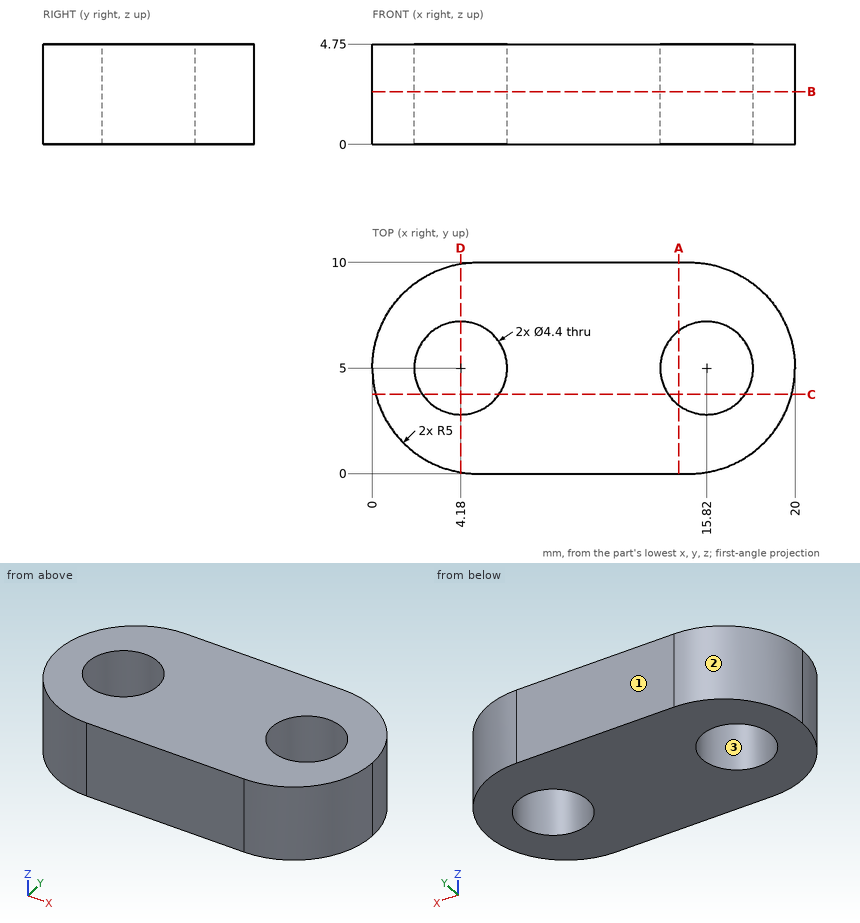
Here's the drawing with two shaded views (mm, measured from the low corner). I have some questions. Round coordinates to 2 decimals unless told otherwise and drop trailing zeros. Write each loop counter-clockwise with the first axis right and the second up, starting at its lowest first coordinate (ties: lowest second). Pieces come first, ordered by that corner, then holes. Notation, with made-up numbers: M 23,-28.75 L 59,-28.75 A28 cw 59,1.25 Z; hole C 41,61.5 d6. An arc over 180 degrees is marked long. Answer in a Markdown table with one row per item. Add a question column.
Q1. Imagine slicing it at B-B (z = 2.5). Give the number of separate pieces and of enclosed holes in the cut face, then the cut area to 3 significant figures.
Q2. If we mould it in two halves opening along X, with no side actions, what happens to the marked faces 1, 2 and 3? For each: +X half, -X half, draft (parallel to the pull), parting line (faces both ways), or undercut.
Q3. Imagine slicing it at A-A (x = 14.5). Please give me the cut outline in (y, z), then the cut area to 3 significant figures.
Q4. If I drill on line 1 (X direction, y = 6, z = 0.55); line 2 (X direction, y = 3.25, z = 2.9); line 3 (Y direction, x = 15.82, z = 3), over which ranges is the centre line in solid material (lowest first)? Write a range as from..to.
Q5. Imagine slicing it at C-C (y = 3.75). Please give me the cut outline in (x, z).
Q6. Imagine slicing it at D-D (x = 4.18). Please give me the cut outline in (y, z), then the cut area to 3 significant figures.
Values:
| question | item | result |
|---|---|---|
| 1 | separate pieces | 1 |
| 1 | enclosed holes | 2 |
| 1 | area | 148 mm^2 |
| 2 | face 1 | draft |
| 2 | face 2 | -X half |
| 2 | face 3 | undercut |
| 3 | outline | M 0,0 L 3.24,0 L 3.24,4.75 L 0,4.75 Z; M 6.76,0 L 10,0 L 10,4.75 L 6.76,4.75 Z |
| 3 | area | 30.8 mm^2 |
| 4 | line 1 | 0.1..2.22, 6.14..13.86, 17.78..19.9 |
| 4 | line 2 | 0.32..2.85, 5.51..14.49, 17.15..19.68 |
| 4 | line 3 | 0.07..2.8, 7.2..9.93 |
| 5 | outline | M 0.16,0 L 2.37,0 L 2.37,4.75 L 0.16,4.75 Z; M 5.99,0 L 14.01,0 L 14.01,4.75 L 5.99,4.75 Z; M 17.63,0 L 19.84,0 L 19.84,4.75 L 17.63,4.75 Z |
| 6 | outline | M 0.07,0 L 2.8,0 L 2.8,4.75 L 0.07,4.75 Z; M 7.2,0 L 9.93,0 L 9.93,4.75 L 7.2,4.75 Z |
| 6 | area | 26.0 mm^2 |
